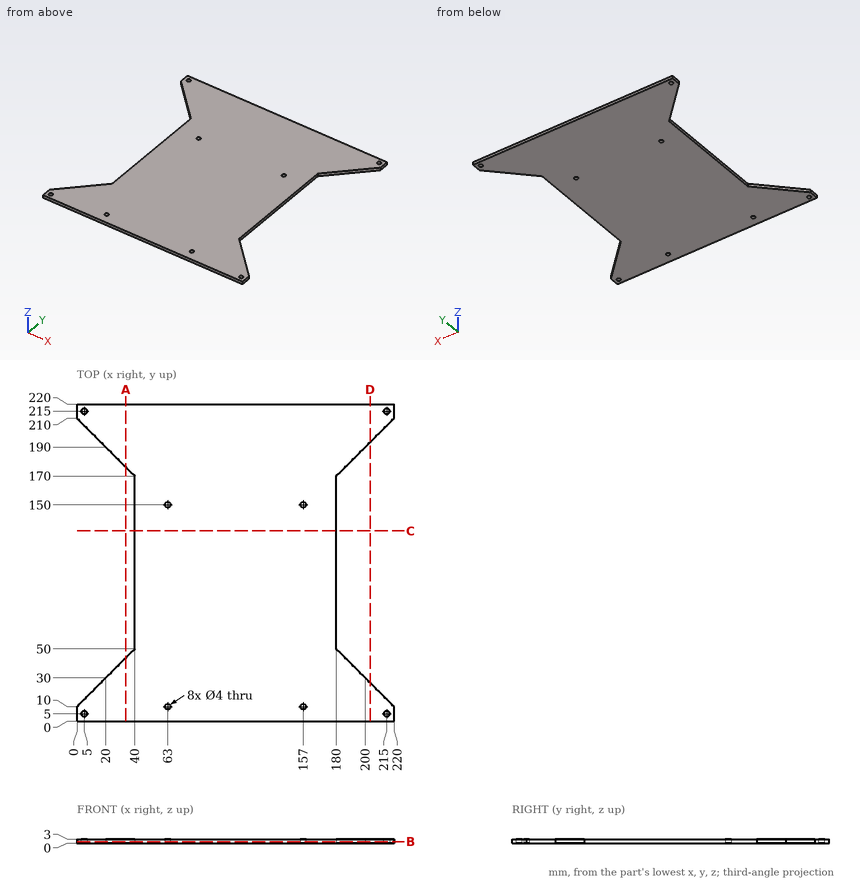
Geometry: see drawing. Coordinates: mm, zero at the bounding-box minimum. Coordinates: 2 decimals unless noted, no trailing zeros. Loops run counter-clockwise (first coordinate to the right, second up) from the corner with the lowest first, then second, coordinate; pieces in that order, holes last. Notation, with made-up numbers: M 6.5,-13.5 L 21.5,-13.5 A23 cw 21.5,12.5 Z; hole C -18,89 d1. An arc over 180 degrees is marked long. Answer in a Markdown table with one row per item.
1. Section A-A, the plane x = 34. Output: boundary loops of the cut face in (y, z), then the cut area to 3 significant figures.
Response:
| item | result |
|---|---|
| outline | M 0,0 L 44,0 L 44,3 L 0,3 Z; M 176,0 L 220,0 L 220,3 L 176,3 Z |
| area | 264 mm2 |
2. Section D-D, the plane x = 203.5. Output: boundary loops of the cut face in (y, z), then the cut area to 3 significant figures.
Response:
| item | result |
|---|---|
| outline | M 0,0 L 26.5,0 L 26.5,3 L 0,3 Z; M 193.5,0 L 220,0 L 220,3 L 193.5,3 Z |
| area | 159 mm2 |
3. Material intervals for line 1 (X direction, y = 215, z = 1); line 2 (Y direction, x = 63, z = 1.75); line 3 (Y direction, x = 215, z = 2.1), sorted ascending.
Response:
| item | result |
|---|---|
| line 1 | x = 0 to 3, 7 to 213, 217 to 220 |
| line 2 | y = 0 to 8, 12 to 148, 152 to 220 |
| line 3 | y = 0 to 3, 7 to 15, 205 to 213, 217 to 220 |
4. Section B-B, the plane z = 1.2. Count the separate pieces of the cut face and the enclosed holes in it, then the cut area to 3 significant figures.
Response:
| item | result |
|---|---|
| separate pieces | 1 |
| enclosed holes | 8 |
| area | 35,500 mm2 |
5. First-contact query: pin 1 (4.5 mm diameter, centred on x = 63, y = 150, fed in from +Z); pin 2 (3.5 mm diameter, centred on x = 5, y = 5, fed in from -Z); pin 3 (1.5 mm diameter, centred on y = 57, z = 0.5, fed in from -X); pin 4 (1 mm diameter, centred on y = 134.5, z = 2, fed in from +X). Flat tips, straight axial feed; report the tip coordinate or a pass-through.
Response:
| item | result |
|---|---|
| pin 1 | stops at z = 3 |
| pin 2 | passes through |
| pin 3 | stops at x = 40 |
| pin 4 | stops at x = 180 |
6. Section C-C, the plane y = 132. Output: boundary loops of the cut face in (x, z).
Response:
| item | result |
|---|---|
| outline | M 40,0 L 180,0 L 180,3 L 40,3 Z |
